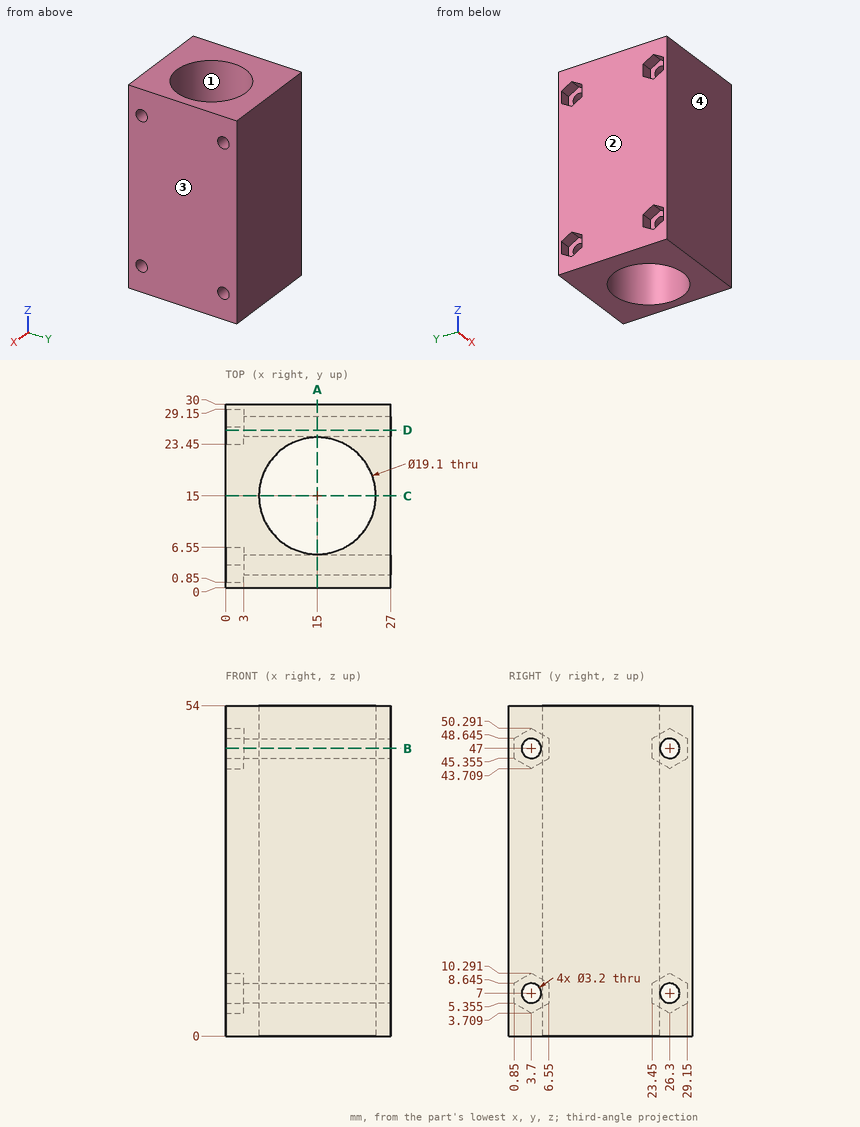
Study the drawing (mm; zero at the part's minimum x, y, z) and answer. Round coordinates to 2 decimals unless told otherwise and drop trailing zeros. Write each loop counter-clockwise with the first axis right and the second up, starting at its lowest first coordinate (ties: lowest second). Pieces come first, ordered by that corner, then holes.
1) A cutting plane is placed at C-C (y = 15). Give the vertices of the cut face in (x, z).
2) The mould has two halves that part along X. Classify the marked faces 1, 2, 3 and 4: pulls with the +X half, pulls with the -X half, needs draft (parallel to the pull), parting line crosses it, or undercut.
3) A cutting plane is placed at B-B (z = 47). Give the vertices of the cut face in (x, y).
4) A cutting plane is placed at A-A (x = 15). Give the vertices of the cut face in (y, z).
5) Straight lines are drawn through the part: line 1 (Z direction, x = 18, y = 3.7); line 2 (X direction, y = 7.5, z = 34) (1 decimal); line 3 (X direction, y = 18, z = 40). For each, find the intervals that lie inside material, in ascending order.
6) Given pin 1 Ø2.5 at (x, z) = (2, 47.5) entering from -Y; pin 2 Ø2.5 at (y, z) = (3.7, 47) entering from +X; pin 3 Ø1.7 at (y, z) = (27.5, 46.5) entering from -X, each flat-ended and moving along its own axis, determine where each tip first touches the part or whether it passes through.
7) A cutting plane is placed at D-D (y = 25.75). Give the vertices of the cut face in (x, z).
Completed:
1. outline: (0, 0) - (5.45, 0) - (5.45, 54) - (0, 54) - close; (24.55, 0) - (27, 0) - (27, 54) - (24.55, 54) - close
2. face 1: undercut
2. face 2: pulls with the -X half
2. face 3: pulls with the +X half
2. face 4: needs draft
3. outline: (0, 0) - (27, 0) - (27, 2.1) - (3, 2.1) - (3, 0.85) - (0, 0.85) - close; (0, 6.55) - (3, 6.55) - (3, 5.3) - (27, 5.3) - (27, 24.7) - (3, 24.7) - (3, 23.45) - (0, 23.45) - close; (0, 29.15) - (3, 29.15) - (3, 27.9) - (27, 27.9) - (27, 30) - (0, 30) - close; hole circle Ø19.1 at (15, 15)
4. outline: (0, 0) - (5.45, 0) - (5.45, 54) - (0, 54) - close; (24.55, 0) - (30, 0) - (30, 54) - (24.55, 54) - close; hole circle Ø3.2 at (3.7, 7); hole circle Ø3.2 at (3.7, 47); hole circle Ø3.2 at (26.3, 7); hole circle Ø3.2 at (26.3, 47)
5. line 1: z = 0 to 5.4, 8.6 to 45.4, 48.6 to 54
5. line 2: x = 0 to 9.1, 20.9 to 27
5. line 3: x = 0 to 5.93, 24.07 to 27
6. pin 1: stops at y = 0
6. pin 2: passes through
6. pin 3: stops at x = 3
7. outline: (0, 0) - (27, 0) - (27, 5.5) - (3, 5.5) - (3, 4.03) - (0, 4.03) - close; (0, 9.97) - (3, 9.97) - (3, 8.5) - (27, 8.5) - (27, 45.5) - (3, 45.5) - (3, 44.03) - (0, 44.03) - close; (0, 49.97) - (3, 49.97) - (3, 48.5) - (27, 48.5) - (27, 54) - (0, 54) - close
